The listing builds one solid part. Answer for the finished solid, in the listing's coordinates (mm). Face numbers are marked on the shaded views. A direction names the side the tool comes from. Coordinates: 2 decimals unless noted, no trailing zeros. Loops run counter-clockwise (first coordinate to the right, second up) from the corner with the lowest first, then second, coordinate; pieces in that order, holes last. Notation, with made-up numbers: (-6.75, 81.5) -> (25.25, 81.5) arc R10 cw to (25.25, 96.5) -> close; hole circle Ø7 at (71, 66). An arc over 180 degrees is marked (long way). Answer in a Markdown table with one row per item.
```python
from build123d import *

# Parameters (mm, degrees)
F0_W     = 914.4
F0_H     = 1219.2
F1_DEPTH = 457.2
F2_T     = -2.54


with BuildPart() as f1:
    # F0 (on Front) → F1 (new body, symmetric)
    with BuildSketch(Plane.XZ):
        Rectangle(F0_W, F0_H)
    extrude(amount=F1_DEPTH, both=True)

    # F2
    f2_openings = [f1.faces().sort_by_distance(p)[0] for p in [
        (0, 0, 609.6),
    ]]
    offset(amount=F2_T, openings=f2_openings)


solid = f1.part
```
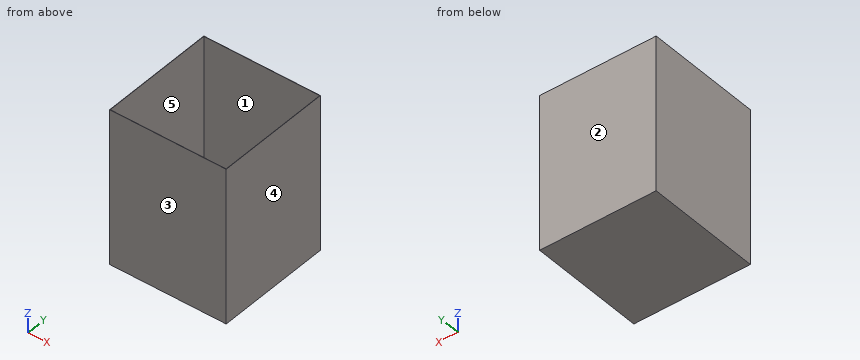
Item 1: Find the intervals of material crossed by probe 1 along X at (y, z) = (-63.5, 538.5); probe 2 along Z at (x, y) = (405, 278), in increasing order.
Findings below:
| item | result |
|---|---|
| probe 1 | x = -457.2 to -454.66, 454.66 to 457.2 |
| probe 2 | z = -609.6 to -607.06 |
Item 2: Determine the mould class of the marked faces 1, 2 and 3 for opening direction Y: +Y half, -Y half, draft (parallel to the pull), parting line (faces both ways), or undercut.
Findings below:
| item | result |
|---|---|
| face 1 | undercut |
| face 2 | +Y half |
| face 3 | -Y half |
Item 3: A tool of negligible diameter and unlimited length cuts with its end or side. For the marked faces 4 and 5, from which of +Z, -Z, +X, -X, +Y, -Y can it reach the whole face along a straight path? Write none if from no direction.
Findings below:
| item | result |
|---|---|
| face 4 | +Z, -Z, +X, +Y, -Y |
| face 5 | +Z |
Item 4: A cutting plane is placed at A-A, the plane z = 452.5. Determine the outline of the cut face in (x, y), plus the area to 3 significant figures.
Findings below:
| item | result |
|---|---|
| outline | (-457.2, -457.2) -> (457.2, -457.2) -> (457.2, 457.2) -> (-457.2, 457.2) -> close; hole (-454.66, -454.66) -> (454.66, -454.66) -> (454.66, 454.66) -> (-454.66, 454.66) -> close |
| area | 9,260 mm2 |
Item 5: A cutting plane is placed at B-B, the plane x = 232.5. Determine the outline of the cut face in (y, z), plus the area to 3 significant figures.
Findings below:
| item | result |
|---|---|
| outline | (-457.2, -609.6) -> (457.2, -609.6) -> (457.2, 609.6) -> (454.66, 609.6) -> (454.66, -607.06) -> (-454.66, -607.06) -> (-454.66, 609.6) -> (-457.2, 609.6) -> close |
| area | 8,500 mm2 |
